Input: part model. Units: mm. Frame: model coordinates. A direction names the side the tool comes from. Round coordinates to 2 decimals unless told otherwise and drop trailing zeros. Loops run counter-clockwise (first coordinate to the right, second up) from the corner with the lowest first, then second, coordinate; pieces in that order, holes last.
(1) Access query for faces 1 (the face through (-44, -29.496, 12)), 2 (the face through (21, -29.496, 12)), 3 (the face through (6, 26.505, 12)). Directions: +Z, -Z, +X, -X, +Y, -Y. A direction counts if a zero-diameter tool reaches every point of the face in a straight line with its end or side. Return the directions, or none.
(2) Cut plane B-B, the plane y = 24.5. Output: boundary loops of the cut face in (x, z), and give its area (3 significant figures).
(3) Cut plane A-A, the plane z = 8.5. Output: boundary loops of the cut face in (x, y), and give its area (3 significant figures).
(4) First-contact query: pin 1 Ø4 at (x, y) = (-2.5, -23) entering from -Z; pin 2 Ø7 at (y, z) = (21, 6.5) entering from -X; pin 3 Ø7 at (x, z) = (22, 9.5) entering from +Y; pin 4 Ø12 at (y, z) = (39, 17.5) entering from -X. Flat tips, straight axial feed; report the tip coordinate or a pass-through.
(5) Line query: line 1 (X direction, y = 14, z = 11); line 2 (X direction, y = 34, z = 18.75); line 3 (Y direction, x = -42.5, z = 2.75). Output: solid intervals per line, ascending.
(6) Cut plane C-C, the plane x = -42. Output: boundary loops of the cut face in (y, z).
from build123d import *

# Parameters (mm, degrees)
F1_DEPTH = 25


with BuildPart() as f1:
    # F0 (on Top) → F1 (new body)
    with BuildSketch(Plane.XY):
        with BuildLine():
            ThreePointArc((-49.571264, -40.496381), (-48.692584, -42.617702), (-46.571264, -43.496381))
            Line((-46.571264, -43.496381), (-39.571264, -43.496381))
            Line((-39.571264, -43.496381), (-27.571264, -43.496381))
            Line((-27.571264, -43.496381), (-11.571264, -43.496381))
            Line((-11.571264, -43.496381), (-11.571264, 12.504975))
            Line((-11.571264, 12.504975), (-28.604711, 12.504975))
            Line((-28.604711, 12.504975), (-34.020273, 12.504975))
            Line((-34.020273, 12.504975), (-39.571264, -29.496381))
            Line((-39.571264, -29.496381), (-48.071264, -29.496381))
            ThreePointArc((-48.071264, -29.496381), (-49.131924, -29.935721), (-49.571264, -30.996381))
            Line((-49.571264, -30.996381), (-49.571264, -40.496381))
        make_face()
        with BuildLine():
            Line((-11.571264, 12.504975), (-11.571264, -43.496381))
            Line((-11.571264, -43.496381), (4.428736, -43.496381))
            Line((4.428736, -43.496381), (16.428736, -43.496381))
            Line((16.428736, -43.496381), (23.428736, -43.496381))
            ThreePointArc((23.428736, -43.496381), (25.550056, -42.617702), (26.428736, -40.496381))
            Line((26.428736, -40.496381), (26.428736, -30.996381))
            ThreePointArc((26.428736, -30.996381), (25.989396, -29.935721), (24.928736, -29.496381))
            Line((24.928736, -29.496381), (16.428736, -29.496381))
            Line((16.428736, -29.496381), (10.877745, 12.504975))
            Line((10.877745, 12.504975), (3.395289, 12.504975))
            Line((3.395289, 12.504975), (-11.571264, 12.504975))
        make_face()
        with BuildLine():
            Line((-28.604711, 12.504975), (-11.571264, 12.504975))
            Line((-11.571264, 12.504975), (-11.571264, 61.503619))
            Line((-11.571264, 61.503619), (-26.229704, 61.503619))
            ThreePointArc((-26.229704, 61.503619), (-27.21844, 61.131626), (-27.716773, 60.200153))
            Line((-27.716773, 60.200153), (-32.170002, 26.504975))
            Line((-32.170002, 26.504975), (-28.604711, 26.504975))
            Line((-28.604711, 26.504975), (-28.604711, 12.504975))
        make_face()
        Polygon((-11.571264, 61.503619), (-11.571264, 12.504975), (3.395289, 12.504975), (3.395289, 26.504975), (3.087176, 61.503619), align=None)
        with BuildLine():
            ThreePointArc((4.574245, 60.200153), (4.075913, 61.131626), (3.087176, 61.503619))
            Line((3.087176, 61.503619), (3.395289, 26.504975))
            Line((3.395289, 26.504975), (9.027474, 26.504975))
            Line((9.027474, 26.504975), (4.574245, 60.200153))
        make_face()
    extrude(amount=F1_DEPTH)


solid = f1.part
Reported:
1. face 1: +Z, -Z, -X, +Y
1. face 2: +Z, -Z, +X, +Y
1. face 3: +Z, -Z, +X
2. outline: (-28.6, 0) - (3.4, 0) - (3.4, 25) - (-28.6, 25) - close
2. area: 800 mm2
3. outline: (-49.57, -40.5) arc R3 ccw to (-46.57, -43.5) - (23.43, -43.5) arc R3 ccw to (26.43, -40.5) - (26.43, -31) arc R1.5 ccw to (24.93, -29.5) - (16.43, -29.5) - (10.88, 12.5) - (3.4, 12.5) - (3.4, 26.5) - (9.03, 26.5) - (4.57, 60.2) arc R1.5 ccw to (3.09, 61.5) - (-26.23, 61.5) arc R1.5 ccw to (-27.72, 60.2) - (-32.17, 26.5) - (-28.6, 26.5) - (-28.6, 12.5) - (-34.02, 12.5) - (-39.57, -29.5) - (-48.07, -29.5) arc R1.5 ccw to (-49.57, -31) - close
3. area: 4,910 mm2
4. pin 1: stops at z = 0
4. pin 2: stops at x = -28.6
4. pin 3: stops at y = -29.5
4. pin 4: stops at x = -31.31
5. line 1: x = -28.6 to 3.4
5. line 2: x = -31.18 to 8.04
5. line 3: y = -43.5 to -29.5
6. outline: (-43.5, 0) - (-29.5, 0) - (-29.5, 25) - (-43.5, 25) - close
